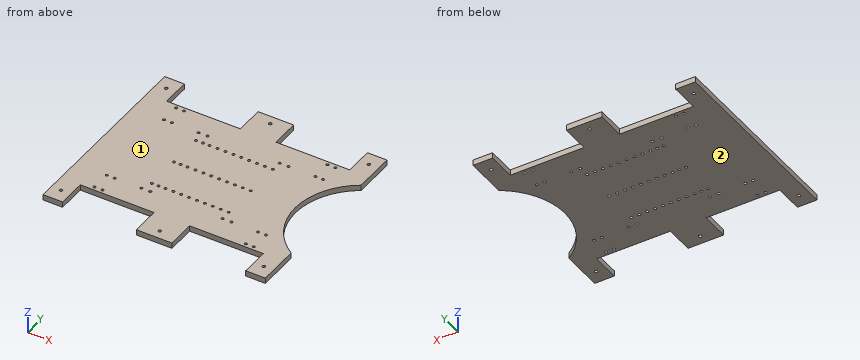
```python
from build123d import *

# Parameters (mm, degrees)
SKETCH1_R           = 1.7525
SKETCH1_R_2         = 1.5
BOSS_EXTRUDE1_DEPTH = 6.35
SKETCH3_R           = 1.5
CUT_EXTRUDE2_DEPTH  = 10


with BuildPart() as part:
    # Sketch1 → Boss-Extrude1 (new body)
    with BuildSketch(Plane.XY):
        with BuildLine():
            Line((119.609790965, 110), (97.609790965, 110))
            Line((97.609790965, 110), (97.609790965, 78))
            Line((97.609790965, 78), (14.609790965, 78))
            Line((14.609790965, 78), (14.609790965, 110))
            Line((14.609790965, 110), (-25.390209035, 110))
            Line((-25.390209035, 110), (-25.390209035, 78))
            Line((-25.390209035, 78), (-108.390209035, 78))
            Line((-108.390209035, 78), (-108.390209035, 110))
            Line((-108.390209035, 110), (-130.390209035, 110))
            Line((-130.390209035, 110), (-130.390209035, -110))
            Line((-130.390209035, -110), (-108.390209035, -110))
            Line((-108.390209035, -110), (-108.390209035, -78))
            Line((-108.390209035, -78), (-25.390209035, -78))
            Line((-25.390209035, -78), (-25.390209035, -110))
            Line((-25.390209035, -110), (14.609790965, -110))
            Line((14.609790965, -110), (14.609790965, -78))
            Line((14.609790965, -78), (97.609790965, -78))
            Line((97.609790965, -78), (97.609790965, -110))
            Line((97.609790965, -110), (119.609790965, -110))
            Line((119.609790965, -110), (119.609790965, -63.2))
            ThreePointArc((119.609790965, -63.2), (84.992460515, 0), (119.609790965, 63.2))
            Line((119.609790965, 63.2), (119.609790965, 110))
        make_face()
        with Locations((-119.390209035, 95)):
            Circle(SKETCH1_R, mode=Mode.SUBTRACT)
        with Locations(Location((108.609790965, 95, 0), (0, 0, 180))):
            Circle(SKETCH1_R, mode=Mode.SUBTRACT)
        with Locations((-5.390209035, 100)):
            Circle(SKETCH1_R, mode=Mode.SUBTRACT)
        with Locations(Location((-5.390209035, -100, 0), (0, 0, 180))):
            Circle(SKETCH1_R, mode=Mode.SUBTRACT)
        with Locations((108.609790965, -95)):
            Circle(SKETCH1_R, mode=Mode.SUBTRACT)
        with Locations(Location((-119.390209035, -95, 0), (0, 0, 180))):
            Circle(SKETCH1_R, mode=Mode.SUBTRACT)
        with Locations((-36.311771099, 40)):
            Circle(SKETCH1_R_2, mode=Mode.SUBTRACT)
        with Locations((-36.311771099, 0)):
            Circle(SKETCH1_R_2, mode=Mode.SUBTRACT)
        with Locations(Location((-36.311771099, -40, 0), (0, 0, 180))):
            Circle(SKETCH1_R_2, mode=Mode.SUBTRACT)
        with Locations(Location((-27.421771099, -40, 0), (0, 0, 180))):
            Circle(SKETCH1_R_2, mode=Mode.SUBTRACT)
        with Locations((-27.421771099, 0)):
            Circle(SKETCH1_R_2, mode=Mode.SUBTRACT)
        with Locations((-27.421771099, 40)):
            Circle(SKETCH1_R_2, mode=Mode.SUBTRACT)
        with Locations(Location((-18.531771099, -40, 0), (0, 0, 180))):
            Circle(SKETCH1_R_2, mode=Mode.SUBTRACT)
        with Locations((-18.531771099, 0)):
            Circle(SKETCH1_R_2, mode=Mode.SUBTRACT)
        with Locations((-18.531771099, 40)):
            Circle(SKETCH1_R_2, mode=Mode.SUBTRACT)
        with Locations(Location((-9.641771099, -40, 0), (0, 0, 180))):
            Circle(SKETCH1_R_2, mode=Mode.SUBTRACT)
        with Locations((-9.641771099, 0)):
            Circle(SKETCH1_R_2, mode=Mode.SUBTRACT)
        with Locations((-9.641771099, 40)):
            Circle(SKETCH1_R_2, mode=Mode.SUBTRACT)
        with Locations(Location((-0.751771099, -40, 0), (0, 0, 180))):
            Circle(SKETCH1_R_2, mode=Mode.SUBTRACT)
        with Locations((-0.751771099, 0)):
            Circle(SKETCH1_R_2, mode=Mode.SUBTRACT)
        with Locations((-0.751771099, 40)):
            Circle(SKETCH1_R_2, mode=Mode.SUBTRACT)
        with Locations(Location((8.138228901, -40, 0), (0, 0, 180))):
            Circle(SKETCH1_R_2, mode=Mode.SUBTRACT)
        with Locations((8.138228901, 0)):
            Circle(SKETCH1_R_2, mode=Mode.SUBTRACT)
        with Locations((8.138228901, 40)):
            Circle(SKETCH1_R_2, mode=Mode.SUBTRACT)
        with Locations(Location((17.028228901, -40, 0), (0, 0, 180))):
            Circle(SKETCH1_R_2, mode=Mode.SUBTRACT)
        with Locations((17.028228901, 0)):
            Circle(SKETCH1_R_2, mode=Mode.SUBTRACT)
        with Locations((17.028228901, 40)):
            Circle(SKETCH1_R_2, mode=Mode.SUBTRACT)
        with Locations(Location((25.918228901, -40, 0), (0, 0, 180))):
            Circle(SKETCH1_R_2, mode=Mode.SUBTRACT)
        with Locations((25.918228901, 0)):
            Circle(SKETCH1_R_2, mode=Mode.SUBTRACT)
        with Locations((25.918228901, 40)):
            Circle(SKETCH1_R_2, mode=Mode.SUBTRACT)
        with Locations(Location((34.808228901, -40, 0), (0, 0, 180))):
            Circle(SKETCH1_R_2, mode=Mode.SUBTRACT)
        with Locations((34.808228901, 0)):
            Circle(SKETCH1_R_2, mode=Mode.SUBTRACT)
        with Locations((34.808228901, 40)):
            Circle(SKETCH1_R_2, mode=Mode.SUBTRACT)
        with Locations((-43.931771099, 0)):
            Circle(SKETCH1_R_2, mode=Mode.SUBTRACT)
        with Locations(Location((-43.931771099, -40, 0), (0, 0, 180))):
            Circle(SKETCH1_R_2, mode=Mode.SUBTRACT)
        with Locations((-43.931771099, 40)):
            Circle(SKETCH1_R_2, mode=Mode.SUBTRACT)
        with Locations((-51.551771099, 0)):
            Circle(SKETCH1_R_2, mode=Mode.SUBTRACT)
        with Locations(Location((-51.551771099, -40, 0), (0, 0, 180))):
            Circle(SKETCH1_R_2, mode=Mode.SUBTRACT)
        with Locations((-51.551771099, 40)):
            Circle(SKETCH1_R_2, mode=Mode.SUBTRACT)
    extrude(amount=BOSS_EXTRUDE1_DEPTH)

    # Sketch3 → Cut-Extrude2 (cut)
    with BuildSketch(Plane.XY.offset(6.35)):
        with Locations((-86.040209035, 73.7)):
            Circle(SKETCH3_R)
        with Locations((-86.040209035, 51.7)):
            Circle(SKETCH3_R)
        with Locations((-56.040209035, 51.7)):
            Circle(SKETCH3_R)
        with Locations(Location((-56.040209035, -51.7, 0), (0, 0, 180))):
            Circle(SKETCH3_R)
        with Locations(Location((-86.040209035, -51.7, 0), (0, 0, 180))):
            Circle(SKETCH3_R)
        with Locations(Location((-86.040209035, -73.7, 0), (0, 0, 180))):
            Circle(SKETCH3_R)
        with Locations((75.259790965, -73.7)):
            Circle(SKETCH3_R)
        with Locations((75.259790965, -51.7)):
            Circle(SKETCH3_R)
        with Locations((45.259790965, -51.7)):
            Circle(SKETCH3_R)
        with Locations(Location((45.259790965, 51.7, 0), (0, 0, 180))):
            Circle(SKETCH3_R)
        with Locations(Location((75.259790965, 51.7, 0), (0, 0, 180))):
            Circle(SKETCH3_R)
        with Locations(Location((75.259790965, 73.7, 0), (0, 0, 180))):
            Circle(SKETCH3_R)
        with Locations((-46.040209035, 51.7)):
            Circle(SKETCH3_R)
        with Locations((-94.890209035, 51.7)):
            Circle(SKETCH3_R)
        with Locations((-94.890209035, 73.7)):
            Circle(SKETCH3_R)
        with Locations(Location((-46.040209035, -51.7, 0), (0, 0, 180))):
            Circle(SKETCH3_R)
        with Locations(Location((-94.890209035, -51.7, 0), (0, 0, 180))):
            Circle(SKETCH3_R)
        with Locations(Location((-94.890209035, -73.7, 0), (0, 0, 180))):
            Circle(SKETCH3_R)
        with Locations(Location((35.259790965, 51.7, 0), (0, 0, 180))):
            Circle(SKETCH3_R)
        with Locations(Location((84.109790965, 51.7, 0), (0, 0, 180))):
            Circle(SKETCH3_R)
        with Locations(Location((84.109790965, 73.7, 0), (0, 0, 180))):
            Circle(SKETCH3_R)
        with Locations((84.109790965, -73.7)):
            Circle(SKETCH3_R)
        with Locations((35.259790965, -51.7)):
            Circle(SKETCH3_R)
        with Locations((84.109790965, -51.7)):
            Circle(SKETCH3_R)
    extrude(amount=-CUT_EXTRUDE2_DEPTH, mode=Mode.SUBTRACT)


solid = part.part
```
Here's how the part is built. I have some questions about the finished solid (model axes, mm). Face numbers are marked on the shaded views. Round coordinates to 2 decimals unless told otherwise and drop trailing zeros. Write each loop counter-clockwise with the first axis right and the second up, starting at its lowest first coordinate (ties: lowest second). Pieces come first, ordered by that corner, then holes.
Q1. Will this pin go through, and if not, where does the flat tip stop? P1, Ø2, axis at x = 47, z = 5.5, coming from the -Y side.
Q2. If we mould it in two halves opening along Z, with no side actions, what happens to the marked faces 1 and 2? For each: +Z half, -Z half, draft (parallel to the pull), parting line (faces both ways), or undercut.
Q3. If we section it at D-D on y = 30: Write out the boundary of the cut face in (x, z).
Q4. If we section it at A-A on y = -89: Write out the boundary of the cut face in (x, z).
Q5. If we section it at C-C on z = 1: Give the number of separate pieces and of enclosed holes in the cut face, plus the area to 3 significant figures.
Q6. If we section it at B-B on x = 90: Write out the boundary of the cut face in (y, z).
Q7. Please list where these lines run through material, in increasing order: probe 1 along X at (y, z) = (81, 4.5); probe 2 along X at (y, z) = (-73.7, 3); probe 3 along Y at (x, z) = (-44.5, 4.5).
Answer below:
1. P1: stops at y = -78
2. face 1: +Z half
2. face 2: -Z half
3. outline: (-130.39, 0) - (91.25, 0) - (91.25, 6.35) - (-130.39, 6.35) - close
4. outline: (-130.39, 0) - (-108.39, 0) - (-108.39, 6.35) - (-130.39, 6.35) - close; (-25.39, 0) - (14.61, 0) - (14.61, 6.35) - (-25.39, 6.35) - close; (97.61, 0) - (119.61, 0) - (119.61, 6.35) - (97.61, 6.35) - close
5. separate pieces: 1
5. enclosed holes: 63
5. area: 40,800 mm2
6. outline: (-78, 0) - (-26.95, 0) - (-26.95, 6.35) - (-78, 6.35) - close; (26.95, 0) - (78, 0) - (78, 6.35) - (26.95, 6.35) - close
7. probe 1: x = -130.39 to -108.39, -25.39 to 14.61, 97.61 to 119.61
7. probe 2: x = -130.39 to -96.39, -93.39 to -87.54, -84.54 to 73.76, 76.76 to 82.61, 85.61 to 119.61
7. probe 3: y = -78 to -41.39, -38.61 to -1.39, 1.39 to 38.61, 41.39 to 78
